from build123d import *

# Parameters (mm, degrees)
ESQUISSE1_W                     = 300
ESQUISSE1_H                     = 200
BOSS_EXTRU_1_DEPTH              = 3
ENL_V_MAT_EXTRU_1_DEPTH         = 10
ESQUISSE3_W                     = 5
ESQUISSE3_H                     = 5
ENL_V_MAT_EXTRU_2_DEPTH         = 10
R_P_TITION_LIN_AIRE1_COUNT      = 2
R_P_TITION_LIN_AIRE1_PITCH      = 75
R_P_TITION_LIN_AIRE1_COUNT_DIR2 = 8
R_P_TITION_LIN_AIRE1_PITCH_DIR2 = 10
ENL_V_MAT_EXTRU_5_DEPTH         = 10
R_P_TITION_LIN_AIRE2_COUNT      = 4
R_P_TITION_LIN_AIRE2_PITCH      = 20
SYM_TRIE1_COPY_1_DEPTH          = 10
SYM_TRIE1_COPY_2_DEPTH          = 10
SYM_TRIE1_COPY_3_DEPTH          = 10
ESQUISSE9_R                     = 1.5
ENL_V_MAT_EXTRU_8_DEPTH         = 10
SYM_TRIE2_COPY_1_DEPTH          = 10
SYM_TRIE2_COPY_2_DEPTH          = 10
SYM_TRIE2_COPY_3_DEPTH          = 10
SYM_TRIE2_COPY_4_DEPTH          = 10
SYM_TRIE2_COPY_5_DEPTH          = 10
SYM_TRIE2_COPY_6_DEPTH          = 10
SYM_TRIE2_COPY_7_DEPTH          = 10
ESQUISSE11_R                    = 11
ESQUISSE11_R_2                  = 3.9
ESQUISSE11_R_3                  = 4.75
ESQUISSE11_R_4                  = 3
ESQUISSE11_R_5                  = 3.95
ENL_V_MAT_EXTRU_10_DEPTH        = 10
ESQUISSE12_W                    = 60
ESQUISSE12_H                    = 60
ENL_V_MAT_EXTRU_11_DEPTH        = 10
ESQUISSE13_W                    = 30
ESQUISSE13_H                    = 60
ENL_V_MAT_EXTRU_12_DEPTH        = 10
ENL_V_MAT_EXTRU_14_DEPTH        = 10
CONG_1_R                        = 10


with BuildPart() as part:
    # Esquisse1 → Boss.-Extru.1 (new body)
    with BuildSketch(Plane(origin=(0, 0, 0), x_dir=(1, 0, 0), z_dir=(0, 1, 0))):
        Rectangle(ESQUISSE1_W, ESQUISSE1_H)
    extrude(amount=BOSS_EXTRU_1_DEPTH)

    # Esquisse2 → Enlèv. mat.-Extru.1 (cut)
    with BuildSketch(Plane(origin=(0, 3, 0), x_dir=(1, 0, 0), z_dir=(0, 1, 0))):
        Polygon((-100, 100), (-150, 50), (-150, 100), align=None)
        Polygon((150, 100), (150, 50), (100, 100), align=None)
        Polygon((150, -100), (150, -50), (100, -100), align=None)
        Polygon((-100, -100), (-150, -100), (-150, -50), align=None)
    extrude(amount=-ENL_V_MAT_EXTRU_1_DEPTH, mode=Mode.SUBTRACT)

    # Esquisse3 → Enlèv. mat.-Extru.2 (cut)
    with BuildSketch(Plane(origin=(0, 3, 0), x_dir=(1, 0, 0), z_dir=(0, 1, 0))):
        with Locations((37.5, -37.5)):
            Rectangle(ESQUISSE3_W, ESQUISSE3_H)
    enl_v_mat_extru_2 = extrude(amount=-ENL_V_MAT_EXTRU_2_DEPTH, mode=Mode.SUBTRACT)

    # Répétition linéaire1: Enl_v. mat.-Extru.2 2 × 8
    with Locations(*[(-i * R_P_TITION_LIN_AIRE1_PITCH, 0, -j * R_P_TITION_LIN_AIRE1_PITCH_DIR2) for i in range(R_P_TITION_LIN_AIRE1_COUNT) for j in range(R_P_TITION_LIN_AIRE1_COUNT_DIR2) if (i, j) != (0, 0)]):
        add(enl_v_mat_extru_2, mode=Mode.SUBTRACT)

    # Esquisse6 → Enlèv. mat.-Extru.5 (cut)
    with BuildSketch(Plane(origin=(0, 3, 0), x_dir=(1, 0, 0), z_dir=(0, 1, 0))):
        Polygon((-142.928932188, 57.071067812), (-150, 50), (-142.928932188, 42.928932188), (-135.857864376, 50), align=None)
    enl_v_mat_extru_5 = extrude(amount=-ENL_V_MAT_EXTRU_5_DEPTH, mode=Mode.SUBTRACT)

    # Répétition linéaire2: Enlèv. mat.-Extru.5 ×4
    with Locations(*[Vector(0.707106781, 0, -0.707106781) * (i * R_P_TITION_LIN_AIRE2_PITCH) for i in range(1, R_P_TITION_LIN_AIRE2_COUNT)]):
        add(enl_v_mat_extru_5, mode=Mode.SUBTRACT)

    # Symétrie1: Enlèv. mat.-Extru.5 across plane
    add(enl_v_mat_extru_5.mirror(Plane.XY), mode=Mode.SUBTRACT)

    # Symétrie1 copy 1 sketch → Symétrie1 copy 1 (cut)
    with BuildSketch(Plane(origin=(14.142135624, 3, 14.142135624), x_dir=(1, 0, 0), z_dir=(0, 1, 0))):
        Polygon((-142.928932188, -57.071067812), (-150, -50), (-142.928932188, -42.928932188), (-135.857864376, -50), align=None)
    extrude(amount=-SYM_TRIE1_COPY_1_DEPTH, mode=Mode.SUBTRACT)

    # Symétrie1 copy 2 sketch → Symétrie1 copy 2 (cut)
    with BuildSketch(Plane(origin=(28.284271247, 3, 28.284271247), x_dir=(1, 0, 0), z_dir=(0, 1, 0))):
        Polygon((-142.928932188, -57.071067812), (-150, -50), (-142.928932188, -42.928932188), (-135.857864376, -50), align=None)
    extrude(amount=-SYM_TRIE1_COPY_2_DEPTH, mode=Mode.SUBTRACT)

    # Symétrie1 copy 3 sketch → Symétrie1 copy 3 (cut)
    with BuildSketch(Plane(origin=(42.426406871, 3, 42.426406871), x_dir=(1, 0, 0), z_dir=(0, 1, 0))):
        Polygon((-142.928932188, -57.071067812), (-150, -50), (-142.928932188, -42.928932188), (-135.857864376, -50), align=None)
    extrude(amount=-SYM_TRIE1_COPY_3_DEPTH, mode=Mode.SUBTRACT)

    # Esquisse9 → Enlèv. mat.-Extru.8 (cut)
    with BuildSketch(Plane(origin=(0, 3, 0), x_dir=(1, 0, 0), z_dir=(0, 1, 0))):
        with Locations((37.5, -2.5)):
            Circle(ESQUISSE9_R)
    enl_v_mat_extru_8 = extrude(amount=-ENL_V_MAT_EXTRU_8_DEPTH, mode=Mode.SUBTRACT)

    # Symétrie2: Enlèv. mat.-Extru.8, Enlèv. mat.-Extru.5 across plane
    add(enl_v_mat_extru_8.mirror(Plane(origin=(0, 0, 0), x_dir=(0, 0, 1), z_dir=(1, 0, 0))), mode=Mode.SUBTRACT)
    add(enl_v_mat_extru_5.mirror(Plane(origin=(0, 0, 0), x_dir=(0, 0, 1), z_dir=(1, 0, 0))), mode=Mode.SUBTRACT)

    # Symétrie2 copy 1 sketch → Symétrie2 copy 1 (cut)
    with BuildSketch(Plane(origin=(0, 3, 0), x_dir=(-1, 0, 0), z_dir=(0, 1, 0))):
        Polygon((-142.928932188, 57.071067812), (-150, 50), (-142.928932188, 42.928932188), (-135.857864376, 50), align=None)
    extrude(amount=-SYM_TRIE2_COPY_1_DEPTH, mode=Mode.SUBTRACT)

    # Symétrie2 copy 2 sketch → Symétrie2 copy 2 (cut)
    with BuildSketch(Plane(origin=(-14.142135624, 3, 14.142135624), x_dir=(-1, 0, 0), z_dir=(0, 1, 0))):
        Polygon((-142.928932188, 57.071067812), (-150, 50), (-142.928932188, 42.928932188), (-135.857864376, 50), align=None)
    extrude(amount=-SYM_TRIE2_COPY_2_DEPTH, mode=Mode.SUBTRACT)

    # Symétrie2 copy 3 sketch → Symétrie2 copy 3 (cut)
    with BuildSketch(Plane(origin=(-28.284271247, 3, 28.284271247), x_dir=(-1, 0, 0), z_dir=(0, 1, 0))):
        Polygon((-142.928932188, 57.071067812), (-150, 50), (-142.928932188, 42.928932188), (-135.857864376, 50), align=None)
    extrude(amount=-SYM_TRIE2_COPY_3_DEPTH, mode=Mode.SUBTRACT)

    # Symétrie2 copy 4 sketch → Symétrie2 copy 4 (cut)
    with BuildSketch(Plane(origin=(-42.426406871, 3, 42.426406871), x_dir=(-1, 0, 0), z_dir=(0, 1, 0))):
        Polygon((-142.928932188, 57.071067812), (-150, 50), (-142.928932188, 42.928932188), (-135.857864376, 50), align=None)
    extrude(amount=-SYM_TRIE2_COPY_4_DEPTH, mode=Mode.SUBTRACT)

    # Symétrie2 copy 5 sketch → Symétrie2 copy 5 (cut)
    with BuildSketch(Plane(origin=(-14.142135624, 3, -14.142135624), x_dir=(-1, 0, 0), z_dir=(0, 1, 0))):
        Polygon((-142.928932188, -57.071067812), (-150, -50), (-142.928932188, -42.928932188), (-135.857864376, -50), align=None)
    extrude(amount=-SYM_TRIE2_COPY_5_DEPTH, mode=Mode.SUBTRACT)

    # Symétrie2 copy 6 sketch → Symétrie2 copy 6 (cut)
    with BuildSketch(Plane(origin=(-28.284271247, 3, -28.284271247), x_dir=(-1, 0, 0), z_dir=(0, 1, 0))):
        Polygon((-142.928932188, -57.071067812), (-150, -50), (-142.928932188, -42.928932188), (-135.857864376, -50), align=None)
    extrude(amount=-SYM_TRIE2_COPY_6_DEPTH, mode=Mode.SUBTRACT)

    # Symétrie2 copy 7 sketch → Symétrie2 copy 7 (cut)
    with BuildSketch(Plane(origin=(-42.426406871, 3, -42.426406871), x_dir=(-1, 0, 0), z_dir=(0, 1, 0))):
        Polygon((-142.928932188, -57.071067812), (-150, -50), (-142.928932188, -42.928932188), (-135.857864376, -50), align=None)
    extrude(amount=-SYM_TRIE2_COPY_7_DEPTH, mode=Mode.SUBTRACT)

    # Esquisse11 → Enlèv. mat.-Extru.10 (cut)
    with BuildSketch(Plane(origin=(0, 3, 0), x_dir=(1, 0, 0), z_dir=(0, 1, 0))):
        with Locations((-70, 60)):
            Circle(ESQUISSE11_R)
        with Locations((110, -40)):
            Circle(ESQUISSE11_R_2)
        with Locations((90, -60)):
            Circle(ESQUISSE11_R_3)
        with Locations((70.071466061, -75.094818152)):
            Circle(ESQUISSE11_R_4)
        with Locations((0, 60)):
            Circle(ESQUISSE11_R_5)
    extrude(amount=-ENL_V_MAT_EXTRU_10_DEPTH, mode=Mode.SUBTRACT)

    # Esquisse12 → Enlèv. mat.-Extru.11 (cut)
    with BuildSketch(Plane(origin=(0, 3, 0), x_dir=(1, 0, 0), z_dir=(0, 1, 0))):
        Rectangle(ESQUISSE12_W, ESQUISSE12_H)
    extrude(amount=-ENL_V_MAT_EXTRU_11_DEPTH, mode=Mode.SUBTRACT)

    # Esquisse13 → Enlèv. mat.-Extru.12 (cut)
    with BuildSketch(Plane(origin=(0, 3, 0), x_dir=(1, 0, 0), z_dir=(0, 1, 0))):
        with Locations((-135, -0.001067812)):
            Rectangle(ESQUISSE13_W, ESQUISSE13_H)
        with Locations((135, -0.001067812)):
            Rectangle(ESQUISSE13_W, ESQUISSE13_H)
    extrude(amount=-ENL_V_MAT_EXTRU_12_DEPTH, mode=Mode.SUBTRACT)

    # Esquisse15 → Enlèv. mat.-Extru.14 (cut)
    with BuildSketch(Plane(origin=(0, 3, 0), x_dir=(1, 0, 0), z_dir=(0, 1, 0))):
        Polygon((-111.462680425, -57.424621202), (-104.391612613, -50.353553391), (-100.856078708, -53.889087297), (-107.927146519, -60.960155108), align=None)
        Polygon((107.927146519, -60.960155108), (100.856078708, -53.889087297), (104.391612613, -50.353553391), (111.462680425, -57.424621202), align=None)
        Polygon((111.462680425, 57.424621202), (104.391612613, 50.353553391), (100.856078708, 53.889087297), (107.927146519, 60.960155108), align=None)
        Polygon((-107.927146519, 60.960155108), (-100.856078708, 53.889087297), (-104.391612613, 50.353553391), (-111.462680425, 57.424621202), align=None)
    extrude(amount=-ENL_V_MAT_EXTRU_14_DEPTH, mode=Mode.SUBTRACT)

    # Congé1
    cong_1_edges = [part.edges().sort_by_distance(p)[0] for p in [
        (-150, 1.5, 30.001067812),
        (-150, 1.5, -29.998932188),
        (150, 1.5, 30.001067812),
        (150, 1.5, -29.998932188),
    ]]
    fillet(cong_1_edges, radius=CONG_1_R)


solid = part.part
Read the model definition and answer for the solid it produces. Units are mm, in the model's axes. A direction names the side the tool comes from. Round coordinates to 2 decimals unless told otherwise and drop trailing zeros. Write each loop counter-clockwise with the first axis right and the second up, starting at its lowest first coordinate (ties: lowest second). Pieces come first, ordered by that corner, then holes. Notation, with made-up numbers: (18, 63.25) - (77, 63.25) arc R24 cw to (77, 73.25) - close; hole circle Ø6 at (47.5, 87.5). An arc over 180 degrees is marked (long way). One line per question, with ' | ' between items. Start each with the question number.
1. For a pull along Z with two mould halves and no side action, classify faces 1 (the face through (-139.344, 1.521, 53.486)), 2 (the face through (31, 0, -1)), 3 (the face through (139, 2, -61)), 4 (the face through (125.3, 1.52, -60.56)) as +Z half, -Z half, draft (parallel to the pull), parting line (faces both ways), or undercut.
2. Each of these flat-tipped pins is pushed along its axis until it touches: pin 1 (0.9 mm diameter, centred on y = 1, z = -22, fed in from +X); pin 2 (1 mm diameter, centred on x = -103.5, y = 2.5, fed in from -Z); pin 3 (0.9 mm diameter, centred on y = 1, z = 17.5, fed in from -X). Where does it stop, or does it pass through?
3. Section B-B (x = 90) is taken. Determine the outline of the cut face in (y, z), and give its area (4 significant figures).
4. Section D-D (y = 1.95) is taken. Give the number of separate pieces and of enclosed holes in the cut face, and give its area (3 significant figures).
5. Section C-C (x = -70) is taken. Determine the outline of the cut face in (y, z).
6. Find the intervals of material crossed by probe 1 along X at (y, z) = (1.8, 2.5); probe 2 along Z at (x, y) = (-70, 1.2); probe 3 along X at (y, z) = (2.1, 14), in increasing order. Write a range as [from, to].
7. Section A-A (x = 0) is taken. Determine the outline of the cut face in (y, z).
8. For faces 5 (the face through (-139, 2, 61)), 6 (the face through (97.02, 1.52, 88.84)), 7 (the face through (-146.99, 1.48, -32.85)), determine the directions among +Z, -Z, +X, -X, +Y, -Y from which every point of the face is accessible in a straight line to the end or side of a thin tool.
Filled in:
1) face 1: undercut | face 2: draft | face 3: -Z half | face 4: undercut
2) pin 1: x = 120 | pin 2: z = -88.85 | pin 3: x = -120
3) outline: (0, -100) - (3, -100) - (3, 55.25) - (0, 55.25) - close; (0, 64.75) - (3, 64.75) - (3, 100) - (0, 100) - close | area: 571.5 mm²
4) separate pieces: 1 | enclosed holes: 28 | area: 44,900 mm²
5) outline: (0, -100) - (3, -100) - (3, -71) - (0, -71) - close; (0, -49) - (3, -49) - (3, 100) - (0, 100) - close
6) probe 1: [-120, -39], [-36, -30], [30, 36], [39, 120] | probe 2: [-100, -71], [-49, 100] | probe 3: [-120, -30], [30, 120]
7) outline: (0, -100) - (3, -100) - (3, -63.95) - (0, -63.95) - close; (0, -56.05) - (3, -56.05) - (3, -30) - (0, -30) - close; (0, 30) - (3, 30) - (3, 100) - (0, 100) - close
8) face 5: +Z, -X, +Y, -Y | face 6: +Y, -Y | face 7: -X, +Y, -Y
